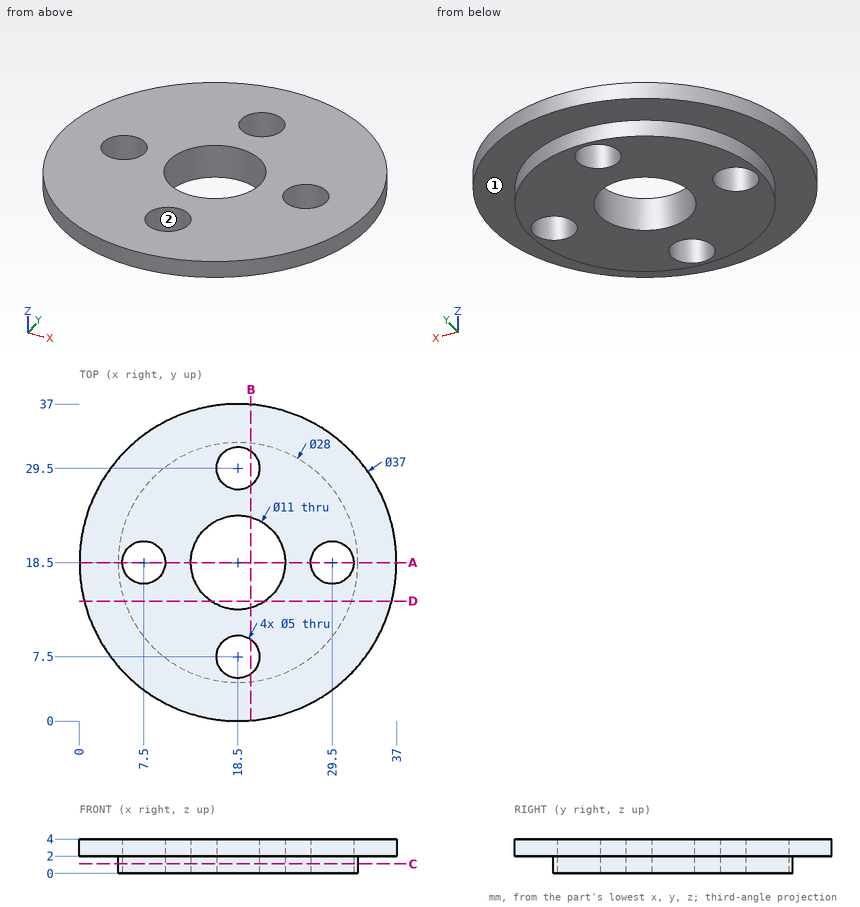
Input: dimensioned drawing with shaded views. Units: mm. Origin: part minimum x, y, z. A direction names the side the tool comes from. Coordinates: 2 decimals unless noted, no trailing zeros. Loops run counter-clockwise (first coordinate to the right, second up) from the corner with the lowest first, then second, coordinate; pieces in that order, holes last. Notation, with made-up numbers: M -21,14.25 L 6,14.25 A16 cw 6,24.25 Z; hole C 65,-37 d11. An arc over 180 degrees is marked long. One line per item, written item: value. Start each with the question number.
1) Material intervals for L1, parallel to Y at x = 18.5, z = 2.9; L2, parallel to Y at x = 18.5, z = 1.15; L3, parallel to Z at x = 35.5, y = 17.5, sorted ascending. Write a range as from..to.
2) Cut plane D-D (y = 14). Return loops of the section in (x, z).
3) Cut plane A-A (y = 18.5). Return loops of the section in (x, z).
4) Cut plane B-B (x = 20). Return loops of the section in (y, z).
5) Cut plane C-C (z = 1.1). Return loops of the section in (x, y).
6) Reachability of the marked faces 1 and 2 from +Z, -Z, +X, -X, +Y, -Y: full face, straight path, thin tool, end or side. Return the list, or none.
7) Pin query (flat end, axial travel): P1, Ø6, axis at x = 18.5, y = 29.5, coming from the -Z side. Return the tip coordinate at first contact, or that it passes through.
Evaluation:
1. L1: 0..5, 10..13, 24..27, 32..37
1. L2: 4.5..5, 10..13, 24..27, 32..32.5
1. L3: 2..4
2. outline: M 0.56,2 L 5.24,2 L 5.24,0 L 15.34,0 L 15.34,4 L 0.56,4 Z; M 21.66,0 L 31.76,0 L 31.76,2 L 36.44,2 L 36.44,4 L 21.66,4 Z
3. outline: M 0,2 L 4.5,2 L 4.5,0 L 5,0 L 5,4 L 0,4 Z; M 10,0 L 13,0 L 13,4 L 10,4 Z; M 24,0 L 27,0 L 27,4 L 24,4 Z; M 32,0 L 32.5,0 L 32.5,2 L 37,2 L 37,4 L 32,4 Z
4. outline: M 0.06,2 L 4.58,2 L 4.58,0 L 5.5,0 L 5.5,4 L 0.06,4 Z; M 9.5,0 L 13.21,0 L 13.21,4 L 9.5,4 Z; M 23.79,0 L 27.5,0 L 27.5,4 L 23.79,4 Z; M 31.5,0 L 32.42,0 L 32.42,2 L 36.94,2 L 36.94,4 L 31.5,4 Z
5. outline: C 18.5,18.5 d28; hole C 7.5,18.5 d5; hole C 18.5,18.5 d11; hole C 18.5,7.5 d5; hole C 18.5,29.5 d5; hole C 29.5,18.5 d5
6. face 1: -Z
6. face 2: +Z, -Z
7. P1: z = 0
